Design review of the part built by this model. Coordinates are the model's own, in mm. A direction names the side the tool comes from. Round coordinates to 2 decimals unless told otherwise and drop trailing zeros. Write each loop counter-clockwise with the first axis right and the second up, starting at its lowest first coordinate (ties: lowest second). Pieces come first, ordered by that corner, then holes.
from build123d import *

# Parameters (mm, degrees)
BOSS_EXTRUDE1_DEPTH = 16
SKETCH2_R           = 2
BOSS_EXTRUDE2_DEPTH = 2
SHELL1_T            = -1
BOSS_EXTRUDE3_REACH = 33.241
SKETCH3_R           = 2.7
SKETCH3_R_2         = 1.7


with BuildPart() as part:
    # Sketch1 → Boss-Extrude1 (new body)
    with BuildSketch(Plane(origin=(0, 0, 0), x_dir=(0, 0, -1), z_dir=(1, 0, 0))):
        Polygon((0, 0), (24, 0), (24, 10), (14.620689655, 10), (0, 2), align=None)
    extrude(amount=BOSS_EXTRUDE1_DEPTH)

    # Sketch2 → Boss-Extrude2 (add)
    with BuildSketch(Plane(origin=(0, 10, 0), x_dir=(1, 0, 0), z_dir=(0, 1, 0))):
        with Locations(Location((4, 20, 0), (0, 0, 90))):
            Circle(SKETCH2_R)
        with Locations(Location((12, 20, 0), (0, 0, 90))):
            Circle(SKETCH2_R)
    extrude(amount=BOSS_EXTRUDE2_DEPTH)

    # Shell1
    shell1_openings = [part.faces().sort_by_distance(p)[0] for p in [
        (8, 0, -12),
    ]]
    offset(amount=SHELL1_T, openings=shell1_openings, kind=Kind.INTERSECTION)

    # Sketch3 → Boss-Extrude3 (add, up to next)
    with BuildSketch(Plane.XZ, mode=Mode.PRIVATE) as boss_extrude3_sk1:
        with Locations(Location((8, -8, 0), (0, 0, 270))):
            Circle(SKETCH3_R)
        with Locations(Location((8, -8, 0), (0, 0, 270))):
            Circle(SKETCH3_R_2, mode=Mode.SUBTRACT)
    boss_extrude3_tool1 = extrude(boss_extrude3_sk1.sketch, amount=-BOSS_EXTRUDE3_REACH, mode=Mode.PRIVATE) - part.part
    # Sketch3 → Boss-Extrude3 (add, up to next)
    with BuildSketch(Plane.XZ, mode=Mode.PRIVATE) as boss_extrude3_sk2:
        with Locations(Location((8, -16, 0), (0, 0, 24.591939532))):
            Circle(SKETCH3_R)
        with Locations(Location((8, -16, 0), (0, 0, 41.372265033))):
            Circle(SKETCH3_R_2, mode=Mode.SUBTRACT)
    boss_extrude3_tool2 = extrude(boss_extrude3_sk2.sketch, amount=-BOSS_EXTRUDE3_REACH, mode=Mode.PRIVATE) - part.part
    add(boss_extrude3_tool1.solids().sort_by_distance((8, 0, -5.376368))[0])
    add(boss_extrude3_tool2.solids().sort_by_distance((5.614345, 0, -17.091832))[0])


solid = part.part
1) For faces 1 (the face through (4, 12, -20)), 2 (the face through (6.966, 2.564, -10.494)), 3 (the face through (5.2, 11, -18.4)), list the 3-axis set-ups (+Z, -Z, +X, -X, +Y, -Y) from which the entire face can be reached by the end or side of a thin tool; tool diameter is ignored.
2) The part is to be moulded in two halves that separate along X. For faces 4 (the face through (10.648, 10.986, -18.526)), 5 (the face through (7.888, 6.056, -7.413)), say which applies: pulls with the +X half, pulls with the -X half, needs draft (parallel to the pull), parting line crosses it, or undercut.
3) For line 1 along X through (y, z) = (3.75, -8); line 2 along X through (y, z) = (9.8, -20); line 3 along X through (y, z) = (5.5, -15.5), list the stretches that pass through material, from the lowest coordinate up.
4) For P1, Ø0.6, axis at x = 12, z = -19.5, coming from the -Y side; P2, Ø3, axis at x = 8, z = -16, coming from the -Y side; P3, Ø1, axis at x = 3.5, z = -7, coming from the +Y side, all flat-tipped, find the tip position at first contact; note any pin that passes through.
5) Add section D-D on x = 1.75. State the section outline as (y, z) points, and give its area (3 significant figures).
6) Add section A-A on y = 4. State the section outline as (x, z) points, and give its area (3 significant figures).
7) Add section C-C on z = -20. State the section outline as (x, y) points.
8) Add section B-B on y = 8. State the section outline as (x, z) points, and give its area (3 significant figures).
Computed:
1. face 1: +Z, -Z, +X, -X, +Y
1. face 2: -Y
1. face 3: +Y
2. face 4: undercut
2. face 5: needs draft
3. line 1: x = 0 to 1, 5.3 to 6.3, 9.7 to 10.7, 15 to 16
3. line 2: x = 0 to 3, 5 to 11, 13 to 16
3. line 3: x = 0 to 1, 5.35 to 6.38, 9.62 to 10.65, 15 to 16
4. P1: stops at y = 11
4. P2: stops at y = 8.79
4. P3: stops at y = 6.1
5. outline: (0, -24) - (10, -24) - (10, -14.62) - (2, 0) - (0, 0) - (0, -1) - (1.41, -1) - (9, -14.88) - (9, -23) - (0, -23) - close
5. area: 36.2 mm2
6. outline: (0, -24) - (16, -24) - (16, -3.66) - (0, -3.66) - close; circle Ø5.4 at (8, -16); hole (1, -23) - (15, -23) - (15, -5.74) - (9.47, -5.74) arc R2.7 cw (long way) to (6.53, -5.74) - (1, -5.74) - close; hole circle Ø3.4 at (8, -16); hole circle Ø3.4 at (8, -8)
6. area: 111 mm2
7. outline: (0, 0) - (1, 0) - (1, 9) - (3, 9) - (3, 11) - (5, 11) - (5, 9) - (11, 9) - (11, 11) - (13, 11) - (13, 9) - (15, 9) - (15, 0) - (16, 0) - (16, 10) - (14, 10) - (14, 12) - (10, 12) - (10, 10) - (6, 10) - (6, 12) - (2, 12) - (2, 10) - (0, 10) - close
8. outline: (0, -24) - (16, -24) - (16, -10.97) - (0, -10.97) - close; circle Ø5.4 at (8, -16); hole (1, -23) - (15, -23) - (15, -13.05) - (1, -13.05) - close; hole circle Ø3.4 at (8, -16)
8. area: 83.1 mm2
